Work out the finished part from the listing and answer in its coordinate system (mm). A direction names the side the tool comes from. Give positions to 0.01 mm unless a question says otherwise; leave off trailing zeros. Write each loop counter-clockwise with the first axis right and the second up, starting at its lowest first coordinate (ties: lowest second). Pieces come first, ordered by that corner, then holes.
1) Find section A-A (y = -291). Determine the outline of the cut face in (x, z) (3 decimals).
2) Find section C-C (z = 23.5). Determine the outline of the cut face in (x, y) (3 decimals).
3) Find section B-B (x = -16). Determine the outline of the cut face in (y, z) (3 decimals), plus the area to 3 significant figures.
4) Given pin 1 Ø21.5 at (x, y) = (-25.5, -187) entering from +Z (3 decimals); pin 2 Ø8 at (x, z) = (-8.5, 23.5) entering from -Y; pin 3 Ø8 at (y, z) = (-288, 21.5) entering from -X (3 decimals), each flat-ended and moving along its own axis, determine where each tip first touches the part or whether it passes through.
5) A tool of negligible diameter and unlimited length cuts with its end or side. For faces 1 (the face through (-11, 0, 2)), 2 (the face through (-3.175, -238, 21)), from which of +Z, -Z, +X, -X, +Y, -Y can it reach the whole face along a straight path? Write none if from no direction.
6) Straight lines are drawn through the part: probe 1 along X at (y, z) = (-325, 32) (3 decimals); probe 2 along Z at (x, y) = (-19, -240) (3 decimals); probe 3 along Z at (x, y) = (-5, -259). For each, find the intervals that lie inside material, in ascending order.
```python
from build123d import *

# Parameters (mm, degrees)
F1_DEPTH = 482.6


with BuildPart() as f1:
    # F0 (on Front) → F1 (new body)
    with BuildSketch(Plane.XZ):
        with BuildLine():
            Line((-3.175, 0), (0, 0))
            Line((0, 0), (0, 3.175))
            Line((0, 3.175), (0, 38.1))
            ThreePointArc((0, 38.1), (-2.374811, 36.431428), (-3.175, 33.641525))
            Line((-3.175, 33.641525), (-3.175, 7.316625))
            ThreePointArc((-3.175, 7.316625), (-4.417453, 4.790697), (-6.722561, 3.175))
            Line((-6.722561, 3.175), (-33.87744, 3.175))
            ThreePointArc((-33.87744, 3.175), (-36.362901, 2.085139), (-38.1, 0))
            Line((-38.1, 0), (-3.175, 0))
        make_face()
    extrude(amount=F1_DEPTH)


solid = f1.part
```
Results:
1. outline: (-38.1, 0) - (0, 0) - (0, 38.1) arc R4.358 ccw to (-3.175, 33.642) - (-3.175, 7.317) arc R5.663 cw to (-6.723, 3.175) - (-33.877, 3.175) arc R5.915 ccw to start
2. outline: (-3.175, -482.6) - (0, -482.6) - (0, 0) - (-3.175, 0) - close
3. outline: (-482.6, 0) - (0, 0) - (0, 3.175) - (-482.6, 3.175) - close
3. area: 1,530 mm2
4. pin 1: stops at z = 3.175
4. pin 2: passes through
4. pin 3: stops at x = -3.175
5. face 1: +Z, -Z, +X, -X, +Y
5. face 2: +Z, -X, +Y, -Y
6. probe 1: x = -3.175 to 0
6. probe 2: z = 0 to 3.175
6. probe 3: z = 0 to 4.2
